```python
from build123d import *

# Parameters (mm, degrees)
SKETCH_1_R               = 10
SKETCH_1_R_2             = 3
SKETCH_1_R_3             = 1.5
EXTRUDE_1_DEPTH          = 8
CUT_EXTRUDE_1_REACH      = 18.248
CUT_EXTRUDE_1_END_RADIUS = 10
SKETCH_2_R               = 1.5
CUT_EXTRUDE_2_REACH      = 18.248
CUT_EXTRUDE_2_END_RADIUS = 10
SKETCH_3_R               = 1.5
CHAMFER_1_SIZE           = 0.5


with BuildPart() as part:
    # ｽｹｯﾁ1 → ﾎﾞｽ - 押し出し1 (new body)
    with BuildSketch(Plane.XY):
        Circle(SKETCH_1_R)
        Circle(SKETCH_1_R_2, mode=Mode.SUBTRACT)
        with Locations((-6, 0)):
            Circle(SKETCH_1_R_3, mode=Mode.SUBTRACT)
        with Locations((6, 0)):
            Circle(SKETCH_1_R_3, mode=Mode.SUBTRACT)
        with Locations((0, 6)):
            Circle(SKETCH_1_R_3, mode=Mode.SUBTRACT)
        with Locations((0, -6)):
            Circle(SKETCH_1_R_3, mode=Mode.SUBTRACT)
    extrude(amount=EXTRUDE_1_DEPTH)

    # ｶｯﾄ - 押し出し1: up to this cylinder (the profile starts inside it)
    cut_extrude_1_end = Plane(origin=(0, 0, 4), z_dir=(0, 0, -1)) * Cylinder(CUT_EXTRUDE_1_END_RADIUS, 57.496, mode=Mode.PRIVATE)
    # ｽｹｯﾁ2 → ｶｯﾄ - 押し出し1 (cut, up to the surface)
    with BuildSketch(Plane(origin=(0, 0, 0), x_dir=(0.7071067811865477, -0.7071067811865475, 0), z_dir=(0.7071067811865475, 0.7071067811865477, 0)), mode=Mode.PRIVATE) as cut_extrude_1_sk1:
        with Locations((0, -4)):
            Circle(SKETCH_2_R)
    cut_extrude_1_tool1 = extrude(cut_extrude_1_sk1.sketch, amount=CUT_EXTRUDE_1_REACH, mode=Mode.PRIVATE) & cut_extrude_1_end
    add(cut_extrude_1_tool1.solids().sort_by_distance((0, 0, 4))[0], mode=Mode.SUBTRACT)

    # ｶｯﾄ - 押し出し2: up to this cylinder (the profile starts inside it)
    cut_extrude_2_end = Plane(origin=(0, 0, 4), z_dir=(0, 0, -1)) * Cylinder(CUT_EXTRUDE_2_END_RADIUS, 57.496, mode=Mode.PRIVATE)
    # ｽｹｯﾁ3 → ｶｯﾄ - 押し出し2 (cut, up to the surface)
    with BuildSketch(Plane(origin=(0, 0, 0), x_dir=(0.7071067811865477, 0.7071067811865475, 0), z_dir=(-0.7071067811865475, 0.7071067811865477, 0)), mode=Mode.PRIVATE) as cut_extrude_2_sk1:
        with Locations(Location((0, -4, 0), (0, 0, 180))):
            Circle(SKETCH_3_R)
    cut_extrude_2_tool1 = extrude(cut_extrude_2_sk1.sketch, amount=-CUT_EXTRUDE_2_REACH, mode=Mode.PRIVATE) & cut_extrude_2_end
    add(cut_extrude_2_tool1.solids().sort_by_distance((0, 0, 4))[0], mode=Mode.SUBTRACT)

    # 面取り1
    chamfer_1_edges = [part.edges().sort_by_distance(p)[0] for p in [
        (-10, 0, 0),
        (-10, 0, 8),
    ]]
    chamfer(chamfer_1_edges, length=CHAMFER_1_SIZE)


solid = part.part
```
Read the model definition and answer for the solid it produces. Units are mm, in the model's axes. Give positions to 0.01 mm unless a question says otherwise; leave off trailing zeros. Write each loop counter-clockwise with the first axis right and the second up, starting at its lowest first coordinate (ties: lowest second). Pieces come first, ordered by that corner, then holes. Notation, with made-up numbers: (8, 17) -> (18, 17) arc R12 ccw to (18, 26) -> close; hole circle Ø9 at (-12, 42.5). An arc over 180 degrees is marked (long way). Answer as a JSON object with one key per item and string values.
1) Straight lines are drawn through the part: probe 1 along Y at (x, z) = (0, 1.75); probe 2 along X at (y, z) = (6.75, 7); probe 3 along X at (y, z) = (-5.5, 6.5). For each, find the intervals that lie inside material, in ascending order. Write a range as from..to.
Findings below:
{"probe 1": "y = -10..-7.5, -4.5..-3, 3..4.5, 7.5..10", "probe 2": "x = -7.38..-1.3, 1.3..7.38", "probe 3": "x = -8.35..-1.41, 1.41..8.35"}
2) Flat-ended cylindrical pins translate along their axes: pin 1 Ø2 at (y, z) = (6, 1) entering from -X; pin 2 Ø3 at (x, z) = (-3.5, 4) entering from +Y. Find the tip coordinate at first contact, or state that the pin passes through.
Findings below:
{"pin 1": "stops at x = -8.66", "pin 2": "stops at y = 9.8"}
3) Section C-C on z = 6.75 is taken. Write down the section's boundary in (x, y).
Findings below:
{"outline": "circle Ø20 at (0, 0); hole circle Ø3 at (-6, 0); hole circle Ø6 at (0, 0); hole circle Ø3 at (0, -6); hole circle Ø3 at (0, 6); hole circle Ø3 at (6, 0)"}
4) For a pull along Z with two mould halves and no side action, classify faces 1 (the cylindrical face through (3.4, -5.4, 4.5)), 2 (the cylindrical face through (-7.2, -0.9, 3.9)), 3 (the flat face through (-2.24, 2.24, 0)), 4 (the cylindrical face through (5.4, 3.4, 3.5)) as pulls with the +Z half, pulls with the -Z half, needs draft (parallel to the pull), parting line crosses it, or undercut.
Findings below:
{"face 1": "undercut", "face 2": "needs draft", "face 3": "pulls with the -Z half", "face 4": "undercut"}
5) Section A-A on y = 0 is taken. Write down the section's boundary in (x, z).
Findings below:
{"outline": "(-10, 0.5) -> (-9.5, 0) -> (-7.5, 0) -> (-7.5, 8) -> (-9.5, 8) -> (-10, 7.5) -> close; (-4.5, 0) -> (-3, 0) -> (-3, 8) -> (-4.5, 8) -> close; (3, 0) -> (4.5, 0) -> (4.5, 8) -> (3, 8) -> close; (7.5, 0) -> (9.5, 0) -> (10, 0.5) -> (10, 7.5) -> (9.5, 8) -> (7.5, 8) -> close"}
6) Section D-D on y = -5.25 is taken. Count the separate pieces of the cut face and the enclosed holes in it, then the cut area to 3 significant figures.
Findings below:
{"separate pieces": "2", "enclosed holes": "1", "area": "105 mm^2"}
